Could you check a few things on this model? Use its own coordinates, in mm. A direction names the side the tool comes from. Give positions to 0.01 mm unless a question says otherwise; leave off trailing zeros. Write each loop counter-clockwise with the first axis right and the second up, starting at its lowest first coordinate (ties: lowest second). Pieces come first, ordered by that corner, then holes. Notation, with made-up numbers: (1.25, -21) - (49.25, -21) arc R23 cw to (49.25, 11) - close; hole circle Ø7 at (32.5, -25.5). An arc over 180 degrees is marked (long way). Answer in a Markdown table with one row per item.
from build123d import *

# Parameters (mm, degrees)
SKETCH1_R           = 12.065
BOSS_EXTRUDE1_DEPTH = 30.988
SKETCH2_R           = 12.446
BOSS_EXTRUDE2_DEPTH = 4.318
SKETCH3_R           = 12.319
BOSS_EXTRUDE3_DEPTH = 14.224
SKETCH4_R           = 12.446
BOSS_EXTRUDE4_DEPTH = 4.318
SKETCH5_R           = 3.5052
BOSS_EXTRUDE5_DEPTH = 2.54
SKETCH6_R           = 1.9812
BOSS_EXTRUDE6_DEPTH = 10.0076
CUT_EXTRUDE1_DEPTH  = 7.9248
SKETCH8_R           = 11.7856
CUT_EXTRUDE2_DEPTH  = 0.889
SKETCH9_R           = 3.175
BOSS_EXTRUDE7_DEPTH = 2.54
FILLET1_R           = 0.762
SKETCH10_R          = 1.397
CUT_EXTRUDE3_DEPTH  = 4.7498


with BuildPart() as part:
    # Sketch1 → Boss-Extrude1 (new body)
    with BuildSketch(Plane(origin=(0, 0, 0), x_dir=(0, 0, -1), z_dir=(1, 0, 0))):
        Circle(SKETCH1_R)
    extrude(amount=BOSS_EXTRUDE1_DEPTH)

    # Sketch2 → Boss-Extrude2 (add)
    with BuildSketch(Plane.ZY):
        Circle(SKETCH2_R)
    extrude(amount=BOSS_EXTRUDE2_DEPTH)

    # Sketch3 → Boss-Extrude3 (add)
    with BuildSketch(Plane.ZY.offset(4.318)):
        Circle(SKETCH3_R)
    extrude(amount=BOSS_EXTRUDE3_DEPTH)

    # Sketch4 → Boss-Extrude4 (add)
    with BuildSketch(Plane.ZY.offset(18.542)):
        Circle(SKETCH4_R)
    extrude(amount=BOSS_EXTRUDE4_DEPTH)

    # Sketch5 → Boss-Extrude5 (add)
    with BuildSketch(Plane.ZY.offset(22.86)):
        Circle(SKETCH5_R)
    extrude(amount=BOSS_EXTRUDE5_DEPTH)

    # Sketch6 → Boss-Extrude6 (add)
    with BuildSketch(Plane.ZY.offset(25.4)):
        Circle(SKETCH6_R)
    extrude(amount=BOSS_EXTRUDE6_DEPTH)

    # Sketch7 → Cut-Extrude1 (cut)
    with BuildSketch(Plane.ZY.offset(35.4076)):
        with BuildLine():
            Line((-1.404828972, 1.397), (1.404828972, 1.397))
            ThreePointArc((1.404828972, 1.397), (0, 1.9812), (-1.404828972, 1.397))
        make_face()
    extrude(amount=-CUT_EXTRUDE1_DEPTH, mode=Mode.SUBTRACT)

    # Sketch8 → Cut-Extrude2 (cut)
    with BuildSketch(Plane(origin=(30.988, 0, 0), x_dir=(0, 0, -1), z_dir=(1, 0, 0))):
        Circle(SKETCH8_R)
    extrude(amount=-CUT_EXTRUDE2_DEPTH, mode=Mode.SUBTRACT)

    # Sketch9 → Boss-Extrude7 (add)
    with BuildSketch(Plane(origin=(30.099, 0, 0), x_dir=(0, 0, -1), z_dir=(1, 0, 0))):
        Circle(SKETCH9_R)
    extrude(amount=BOSS_EXTRUDE7_DEPTH)

    # Fillet1
    fillet1_edges = [part.edges().sort_by_distance(p)[0] for p in [
        (30.099, 0, 3.175),
        (32.639, 0, 3.175),
    ]]
    fillet(fillet1_edges, radius=FILLET1_R)

    # Sketch10 → Cut-Extrude3 (cut)
    with BuildSketch(Plane.ZY.offset(22.86)):
        with Locations((8.509, 0)):
            Circle(SKETCH10_R)
        with Locations((-8.509, 0)):
            Circle(SKETCH10_R)
    extrude(amount=-CUT_EXTRUDE3_DEPTH, mode=Mode.SUBTRACT)


solid = part.part
1) Imagine slicing it at B-B (y = 10). List the corners of the cut face in (x, z) for me, then the cut area to 3 significant figures.
Check values:
| item | result |
|---|---|
| outline | (-22.86, -7.41) - (-18.54, -7.41) - (-18.54, -7.19) - (-4.32, -7.19) - (-4.32, -7.41) - (0, -7.41) - (0, -6.75) - (30.99, -6.75) - (30.99, -6.24) - (30.1, -6.24) - (30.1, 6.24) - (30.99, 6.24) - (30.99, 6.75) - (0, 6.75) - (0, 7.41) - (-4.32, 7.41) - (-4.32, 7.19) - (-18.54, 7.19) - (-18.54, 7.41) - (-22.86, 7.41) - close |
| area | 740 mm2 |
2) Imagine slicing it at C-C (x = 6). List the corners of the cut face in (y, z) for me (3 decimals).
Check values:
| item | result |
|---|---|
| outline | circle Ø24.13 at (0, 0) |
3) Will these pins go through, and if not, where does the flat tip stop? P1, Ø3, axis at y = 0, z = -8.509, coming from the +X side; P2, Ø1.4, axis at y = -0.5, z = 8.5, coming from the -X side; P3, Ø5, axis at y = 0.5, z = -7.5, coming from the -X side.
Check values:
| item | result |
|---|---|
| P1 | stops at x = 30.1 |
| P2 | stops at x = -18.11 |
| P3 | stops at x = -22.86 |
4) Imagine slicing it at A-A (z = 4.75). List the corners of the cut face in (x, y) for me.
Check values:
| item | result |
|---|---|
| outline | (-22.86, -11.5) - (-18.54, -11.5) - (-18.54, -11.37) - (-4.32, -11.37) - (-4.32, -11.5) - (0, -11.5) - (0, -11.09) - (30.99, -11.09) - (30.99, -10.79) - (30.1, -10.79) - (30.1, 10.79) - (30.99, 10.79) - (30.99, 11.09) - (0, 11.09) - (0, 11.5) - (-4.32, 11.5) - (-4.32, 11.37) - (-18.54, 11.37) - (-18.54, 11.5) - (-22.86, 11.5) - close |
5) We'd pull the mould along Y, two halves only. Please class faces 1 (the face through (-22.86, -3, 3)), 2 (the face through (-2.13, -12.15, -2.7)), 3 (the face through (30.55, 3.54, -11.24)): +Y half, -Y half, draft (parallel to the pull), parting line (faces both ways), or undercut.
Check values:
| item | result |
|---|---|
| face 1 | draft |
| face 2 | parting line |
| face 3 | undercut |
6) Imagine slicing it at D-D (x = -3.5). List the corners of the cut face in (y, z) for me, then the cut area to 3 significant figures.
Check values:
| item | result |
|---|---|
| outline | circle Ø24.89 at (0, 0) |
| area | 487 mm2 |
7) If I drill on line 1 (Y direction, x = 30.75, z = 0) (3 decimals); line 2 (Y direction, x = 30.35, z = 0) (3 decimals); line 3 (X direction, y = -1.75, z = -7.5), over which ranges is the centre line in solid material (lowest first)?
Check values:
| item | result |
|---|---|
| line 1 | y = -12.065 to -11.786, -3.183 to 3.183, 11.786 to 12.065 |
| line 2 | y = -12.065 to -11.786, -3.372 to 3.372, 11.786 to 12.065 |
| line 3 | x = -22.86 to 30.1 |
8) On a 3-axis mill with a long thin cutter (end or side, diameter ignored), from which of +Z, -Z, +X, -X, +Y, -Y can I reach the whole of each face in a straight line? I mean faces 4 (the face through (31.36, -3.1, 0.69)), 5 (the face through (-35.408, 0, 0)), 6 (the face through (-32, 1.397, 0)), 7 (the face through (-20.67, -12.15, -2.7)), 8 (the face through (-24.112, 1.053, 3.343)). Say none if no direction works.
Check values:
| item | result |
|---|---|
| face 4 | +X |
| face 5 | +Z, -Z, -X, +Y, -Y |
| face 6 | +Z, -Z, -X, +Y |
| face 7 | +X, -X |
| face 8 | -X |
